The listing builds one solid part. Answer for the finished solid, in the listing's coordinates (mm). A direction names the side the tool comes from. Coordinates: 2 decimals unless noted, no trailing zeros. Order: outer loops, then holes, each group sorted by start corner. A loop starts at its lowest first (then second) coordinate and runs counter-clockwise, first axis right, second up. Notation, with made-up numbers: (0.5, 54) -> (27.5, 54) arc R27 ccw to (27.5, 70) -> close; hole circle Ø10 at (44.5, 0.5). An arc over 180 degrees is marked (long way). Write each question's results on one line, items separated by ' | '. Start each with the question number.
(1) A tool of negligible diameter and unlimited length cuts with its end or side. For faces 1 (the face through (98.493, -33.393, 39.44)), 2 (the face through (87.448, -87.908, 40.56)), from which of +Z, -Z, +X, -X, +Y, -Y can it reach the whole face along a straight path? Write none if from no direction.
(2) Determine the mould class of faces 3 (the face through (-107, 107, 41)), 4 (the face through (110, 2, 39)), 5 (the face through (-110, 5, 39)), 6 (the face through (-87.908, -87.448, 40.56)) for opening direction X: +X half, -X half, draft (parallel to the pull), parting line (faces both ways), or undercut.
(3) The part is cut by section A-A, the plane y = 44. Give the vertices of the cut face in (x, z).
(4) The part is cut by section C-C, the plane x = 17. Give the vertices of the cut face in (y, z), then the cut area to 3 significant figures.
(5) The part is cut by section D-D, the plane x = -32.5. Give the vertices of the cut face in (y, z), then the cut area to 3 significant figures.
(6) The part is cut by section B-B, the plane y = -39. Give the vertices of the cut face in (x, z), then the cut area to 3 significant figures.
(7) Straight lines are drawn through the part: L1, parallel to X at y = 58.5, z = 4; L2, parallel to Y at x = -88, z = 39.5; L3, parallel to X at y = -94, z = 52.5. For each, find the intervals that lie inside material, in ascending order.
```python
from build123d import *

# Parameters (mm, degrees)
BOSS_EXTRUDE1_DEPTH = 80
SKETCH3_R           = 11.5
CUT_EXTRUDE1_DEPTH  = 175.928556845
FILLET1_R           = 3
CHAMFER1_SIZE       = 10
SKETCH4_W           = 220
SKETCH4_H           = 3
CUT_EXTRUDE2_DEPTH  = 175.928557017


with BuildPart() as part:
    # Sketch1 → Boss-Extrude1 (new body)
    with BuildSketch(Plane.XY):
        with BuildLine():
            Line((-104, 0), (-104, 110))
            Line((-104, 110), (-110, 110))
            Line((-110, 110), (-110, -110))
            Line((-110, -110), (110, -110))
            Line((110, -110), (110, 110))
            Line((110, 110), (104, 110))
            Line((104, 110), (104, 0))
            ThreePointArc((104, 0), (0, -104), (-104, 0))
        make_face()
    extrude(amount=BOSS_EXTRUDE1_DEPTH)

    # Sketch3 → Cut-Extrude1 (cut, through all)
    with BuildSketch(Plane.XY.offset(80)):
        with Locations((-79.549512883, -79.549512883)):
            Circle(SKETCH3_R)
        with Locations((79.549512883, -79.549512883)):
            Circle(SKETCH3_R)
    extrude(amount=-CUT_EXTRUDE1_DEPTH, mode=Mode.SUBTRACT)

    # Fillet1
    fillet1_edges = [part.edges().sort_by_distance(p)[0] for p in [
        (-78.613411263, -68.087675607, 40),
        (-68.087675607, -78.613411263, 40),
        (68.087675607, -78.613411263, 40),
        (78.613411263, -68.087675607, 40),
    ]]
    fillet(fillet1_edges, radius=FILLET1_R)

    # Chamfer1
    chamfer1_edges = [part.edges().sort_by_distance(p)[0] for p in [
        (110, -110, 40),
        (-110, -110, 40),
    ]]
    chamfer(chamfer1_edges, length=CHAMFER1_SIZE)

    # Sketch4 → Cut-Extrude2 (cut, through all)
    with BuildSketch(Plane.XY.offset(80)):
        with Locations((0, 108.5)):
            Rectangle(SKETCH4_W, SKETCH4_H)
    extrude(amount=-CUT_EXTRUDE2_DEPTH, mode=Mode.SUBTRACT)


solid = part.part
```
Established:
1) face 1: +Z, -Z, +Y | face 2: +Z, -Z
2) face 3: draft | face 4: +X half | face 5: -X half | face 6: undercut
3) outline: (-110, 0) -> (-104, 0) -> (-104, 80) -> (-110, 80) -> close; (104, 0) -> (110, 0) -> (110, 80) -> (104, 80) -> close
4) outline: (-110, 0) -> (-102.6, 0) -> (-102.6, 80) -> (-110, 80) -> close | area: 592 mm^2
5) outline: (-110, 0) -> (-98.79, 0) -> (-98.79, 80) -> (-110, 80) -> close | area: 897 mm^2
6) outline: (-110, 0) -> (-96.41, 0) -> (-96.41, 80) -> (-110, 80) -> close; (96.41, 0) -> (110, 0) -> (110, 80) -> (96.41, 80) -> close | area: 2,170 mm^2
7) L1: x = -110 to -104, 104 to 110 | L2: y = -110 to -87.35, -71.75 to -55.43 | L3: x = -110 to -44.5, 44.5 to 110
